```python
from build123d import *

# Parameters (mm, degrees)
F0_R     = 14
F0_R_2   = 1.25
F0_R_3   = 3
F0_R_4   = 4.5
F1_DEPTH = 3
F0_R_5   = 1.5
F2_DEPTH = 5


with BuildPart() as f1:
    # F0 (on Top) → F1 (new body)
    with BuildSketch(Plane.XY):
        Circle(F0_R)
        with Locations((-7.7781745931, -7.7781745931)):
            Circle(F0_R_2, mode=Mode.SUBTRACT)
        with Locations((0, -8)):
            Circle(F0_R_3, mode=Mode.SUBTRACT)
        with Locations((7.7781745931, -7.7781745931)):
            Circle(F0_R_2, mode=Mode.SUBTRACT)
        with Locations((-8, 0)):
            Circle(F0_R_3, mode=Mode.SUBTRACT)
        with Locations((-7.7781745931, 7.7781745931)):
            Circle(F0_R_2, mode=Mode.SUBTRACT)
        Circle(F0_R_4, mode=Mode.SUBTRACT)
        with Locations((8, 0)):
            Circle(F0_R_3, mode=Mode.SUBTRACT)
        with Locations((0, 8)):
            Circle(F0_R_3, mode=Mode.SUBTRACT)
        with Locations((7.7781745931, 7.7781745931)):
            Circle(F0_R_2, mode=Mode.SUBTRACT)
    extrude(amount=-F1_DEPTH)

    # F0 (on Top) → F2 (join)
    with BuildSketch(Plane.XY):
        Circle(F0_R)
        with Locations((-7.7781745931, -7.7781745931)):
            Circle(F0_R_2, mode=Mode.SUBTRACT)
        with Locations((0, -8)):
            Circle(F0_R_3, mode=Mode.SUBTRACT)
        with Locations((7.7781745931, -7.7781745931)):
            Circle(F0_R_2, mode=Mode.SUBTRACT)
        with Locations((-8, 0)):
            Circle(F0_R_3, mode=Mode.SUBTRACT)
        with Locations((-7.7781745931, 7.7781745931)):
            Circle(F0_R_2, mode=Mode.SUBTRACT)
        Circle(F0_R_4, mode=Mode.SUBTRACT)
        with Locations((8, 0)):
            Circle(F0_R_3, mode=Mode.SUBTRACT)
        with Locations((0, 8)):
            Circle(F0_R_3, mode=Mode.SUBTRACT)
        with Locations((7.7781745931, 7.7781745931)):
            Circle(F0_R_2, mode=Mode.SUBTRACT)
        with Locations((-8, 0)):
            Circle(F0_R_3)
        with Locations((-8, 0)):
            Circle(F0_R_5, mode=Mode.SUBTRACT)
        with Locations((0, 8)):
            Circle(F0_R_3)
        with Locations((0, 8)):
            Circle(F0_R_5, mode=Mode.SUBTRACT)
        with Locations((8, 0)):
            Circle(F0_R_3)
        with Locations((8, 0)):
            Circle(F0_R_5, mode=Mode.SUBTRACT)
        with Locations((0, -8)):
            Circle(F0_R_3)
        with Locations((0, -8)):
            Circle(F0_R_5, mode=Mode.SUBTRACT)
    extrude(amount=F2_DEPTH)


solid = f1.part
```
Can you work these out from the model? Positions are in its coordinate system, mm. A direction names the side the tool comes from. Give positions to 0.01 mm unless a question says otherwise; leave off trailing zeros. Order: outer loops, then holes, each group sorted by start corner. A loop starts at its lowest first (then second) coordinate and runs counter-clockwise, first axis right, second up. Notation, with made-up numbers: M -29,69.25 L 29,69.25 A9 cw 29,81.25 Z; hole C -7.5,-3.75 d1. An arc over 180 degrees is marked long. One line per item, written item: value.
1) We'd pull the mould along X, two halves only. Please class faces 1 (the face through (-3.3, 3.3, 5)), 2 (the face through (1.61, 10.53, -1.48)): released by +X, released by -X, zero draft, split by the parting line, or undercut.
Answer sheet:
face 1: zero draft
face 2: undercut
2) I want a section at C-C, the plane z = 4.25. Count the separate pieces of the cut face and the enclosed holes in it, plus the area to 3 significant figures.
Answer sheet:
separate pieces: 1
enclosed holes: 9
area: 504 mm^2
3) I want a section at D-D, the plane y = 3.75. List the corners of the cut face in (x, z) for me.
Answer sheet:
outline: M -13.49,-3 L -2.49,-3 L -2.49,5 L -13.49,5 Z; M 2.49,-3 L 13.49,-3 L 13.49,5 L 2.49,5 Z
4) I want a section at A-A, the plane y = 0. List the corners of the cut face in (x, z) for me.
Answer sheet:
outline: M -14,-3 L -11,-3 L -11,0 L -9.5,0 L -9.5,5 L -14,5 Z; M -6.5,0 L -5,0 L -5,-3 L -4.5,-3 L -4.5,5 L -6.5,5 Z; M 4.5,-3 L 5,-3 L 5,0 L 6.5,0 L 6.5,5 L 4.5,5 Z; M 9.5,0 L 11,0 L 11,-3 L 14,-3 L 14,5 L 9.5,5 Z
5) Please list where these lines run through material, in increasing order: line 1 along Y through (x, z) = (0, 1.5); line 2 along Y through (x, z) = (0, -1.45); line 3 along Z through (x, y) = (0.75, -6).
Answer sheet:
line 1: y = -14 to -9.5, -6.5 to -4.5, 4.5 to 6.5, 9.5 to 14
line 2: y = -14 to -11, -5 to -4.5, 4.5 to 5, 11 to 14
line 3: z = 0 to 5
6) For P1, Ø2, axis at y = -2, z = 2.5, coming from the -X side; P2, Ø1.8, axis at x = -6.5, y = 0.5, coming from the -Z side; P3, Ø4, axis at y = -5, z = 3, coming from the +X side, each with a flat end and sliding along its axis, tell me the tip position at first contact or that it passes through.
Answer sheet:
P1: stops at x = -13.96
P2: stops at z = 0
P3: stops at x = 13.67
7) I want a section at B-B, the plane x = 8. List the corners of the cut face in (y, z) for me.
Answer sheet:
outline: M -11.49,-3 L -9.01,-3 L -9.01,5 L -11.49,5 Z; M -6.55,-3 L -3,-3 L -3,0 L -1.5,0 L -1.5,5 L -6.55,5 Z; M 1.5,0 L 3,0 L 3,-3 L 6.55,-3 L 6.55,5 L 1.5,5 Z; M 9.01,-3 L 11.49,-3 L 11.49,5 L 9.01,5 Z
8) On a 3-axis mill with a long thin cutter (end or side, diameter ignored), from which of +Z, -Z, +X, -X, +Y, -Y can I reach the whole of each face in a straight line? I mean faces 3 (the face through (-6.7, -1.3, 0)), 4 (the face through (-3.3, 3.3, -3)). Say none if no direction works.
Answer sheet:
face 3: -Z
face 4: -Z, +X, -X, +Y, -Y
